Autodesk Inventor part; units mm, degrees
ref_plane "YZ Plane" through (0, 0, 0) normal (1, 0, 0) x (0, 1, 0)
ref_plane "XZ Plane" through (0, 0, 0) normal (0, 1, 0) x (-1, 0, 0)
ref_plane "XY Plane" through (0, 0, 0) normal (0, 0, 1) x (1, 0, 0)
sketch "Sketch1" plane through (0, 0, 0) normal (0, 1, 0) x (-1, 0, 0)
  line L0 (0, 0) -> (0, -32)
  line L1 (0, -32) -> (10.9556, -32)
  line L2 (10.9556, -32) -> (10.9556, 0)
  line L3 (10.9556, 0) -> (0, 0)
  dimension "d0" = 32
  dimension "d1" = 10.9556
extrude "Extrusion1" add sketch "Sketch1" along normal blind 2
sketch "Sketch2" plane through (-10.9556, 0, 0) normal (0, 0, 1) x (1, 0, 0)
  line L0 (10.9556, 0) -> (0, 0)
  line L1 (10.9556, 0) -> (9.9556, 0)
  line L2 (9.9556, 0) -> (9.9556, 2)
  line L3 (10.9556, 2) -> (0, 2)
  line L4 (10.9556, 2) -> (9.9556, 0)
  line L5 (0, 0) -> (0, 2)
  line L6 (0, 0) -> (1, 0)
  line L7 (1, 0) -> (0, 2)
  line L8 (1, 0) -> (0, 0)
  line L9 (0, 2) -> (0, 0)
  line L10 (0, 2) -> (10.9556, 2)
  line L11 (9.9556, 0) -> (1, 0)
  line L12 (9.9556, 0) -> (10.9556, 0)
  line L13 (10.9556, 0) -> (10.9556, 2)
  line L14 (10.9556, 2) -> (10.9556, 0)
  line L15 (10.9556, 0) -> (9.9556, 0)
  dimension "d4" = 1
  dimension "d5" = 1
extrude "Extrusion2" cut sketch "Sketch2" against normal through all contours L0 L4 L13 | L0 L5 L7
sketch "Sketch3" plane through (0, 2, 0) normal (0, 1, 0) x (1, 0, 0)
  line L0 (-10.9556, 32) -> (-10.9556, 0)
  line L1 (-10.9556, 32) -> (-10.9556, 0)
  line L2 (-10.9556, 0) -> (-10.9556, 16)
  line L3 (-10.9556, 16) -> (0, 16)
  line L4 (0, 0) -> (0, 32)
  line L5 (-10.9556, 0) -> (0, 0)
  line L6 (0, 32) -> (-10.9556, 32)
  line L7 (-10.9556, 32) -> (-10.9556, 30)
  line L8 (-10.9556, 28.5) -> (0, 28.5)
  line L9 (-10.9556, 0) -> (-10.9556, 2)
  line L10 (-10.9556, 3.5) -> (0, 3.5)
  line L11 (-10.9556, 30) -> (-10.9556, 22)
  line L12 (-10.9556, 20.5) -> (0, 20.5)
  line L13 (-10.9556, 2) -> (-10.9556, 10)
  line L14 (-10.9556, 11.5) -> (0, 11.5)
  line L15 (-10.9556, 20.5) -> (-11.494, 20.5)
  line L16 (-11.494, 20.5) -> (-11.494, 28.5)
  line L17 (-11.494, 28.5) -> (-10.9556, 28.5)
  line L18 (-11.494, 28.5) -> (-13.5464, 28.5)
  line L19 (-13.5464, 28.5) -> (-13.5464, 20.5)
  line L20 (-13.5464, 20.5) -> (-11.494, 20.5)
  line L21 (-11.494, 28.5) -> (-12.994, 28.5)
  line L22 (-11.494, 28.5) -> (-9.994, 28.5)
  line L23 (0, 30) -> (0, 22)
  line L24 (0, 20.5) -> (0.538, 20.5)
  line L25 (0.538, 20.5) -> (0.538, 28.5)
  line L26 (0.538, 28.5) -> (0, 28.5)
  line L27 (0.538, 28.5) -> (2.59, 28.5)
  line L28 (2.59, 28.5) -> (2.59, 20.5)
  line L29 (2.59, 20.5) -> (0.538, 20.5)
  line L30 (0.538, 28.5) -> (2.038, 28.5)
  line L31 (2.038, 28.5) -> (2.038, 20.5)
  line L32 (0.538, 28.5) -> (-0.962, 28.5)
  line L33 (-0.962, 30) -> (-0.962, 22)
  line L34 (-10.9556, 11.5) -> (-11.4936, 11.5)
  line L35 (-11.4936, 11.5) -> (-13.5456, 11.5)
  line L36 (-13.5456, 11.5) -> (-13.5456, 3.5)
  line L37 (-13.5456, 3.5) -> (-10.9556, 3.5)
  line L38 (0, 11.5) -> (0.538, 11.5)
  line L39 (0.538, 11.5) -> (2.59, 11.5)
  line L40 (2.59, 11.5) -> (2.59, 3.5)
  line L41 (2.59, 3.5) -> (0, 3.5)
  line L42 (0, 10) -> (0, 11.5)
  line L43 (0, 11.5) -> (-10.9556, 11.5)
  line L44 (0, 22) -> (0, 20.5)
  dimension "d8" = 32
  dimension "d10" = 2
  dimension "d11" = 2
  dimension "d12" = 8
  dimension "d13" = 8
  dimension "d14" = 0.5384
  dimension "d15" = 2.0524
  dimension "d16" = 1.5
  dimension "d17" = 1.5
  dimension "d23" = 0.538
  dimension "d24" = 2.052
  dimension "d25" = 1.5
  dimension "d26" = 1.5
  dimension "d27" = 0.538
  dimension "d28" = 2.052
  dimension "d29" = 0.538
  dimension "d43" = 1.5
  dimension "d44" = 1.5
extrude "Extrusion3" add sketch "Sketch3" along normal blind 4.4114 contours L8 L4 L12 L0 | L0 L15 L16 L17 | L16 L20 L19 L18 | L26 L25 L24 L4 | L27 L31 L29 L25 | L27 L28 L29 L31 | L14 L4 L10 L0 | L0 L37 L36 L35 L34 | L38 L39 L40 L41 L4
fillet "Fillet1" radius 2.2055 8 edges at (2.59, 6.4114, -7.5) (2.59, 2, -7.5) (2.59, 6.4114, -24.5) (2.59, 2, -24.5) (-13.5464, 6.4114, -24.5) (-13.5464, 2, -24.5) (-13.5456, 6.4114, -7.5) (-13.5456, 2, -7.5)
sketch "Sketch4" plane through (0, 6.4114, 0) normal (0, 1, 0) x (1, 0, 0)
  line L0 (-11.3401, 3.5) -> (-11.3401, 11.5)
  line L1 (-11.3401, 11.5) -> (-11.3401, 3.5)
  line L2 (-11.3401, 3.5) -> (-11.3401, 7.5)
  line L3 (-11.3401, 7.5) -> (-13.5456, 7.5)
  line L4 (-13.5456, 3.5) -> (-13.5456, 11.5)
  line L5 (-11.3401, 7.5) -> (2.59, 7.5)
  line L6 (2.59, 11.5) -> (2.59, 3.5)
  line L7 (0.3845, 3.5) -> (0.3845, 11.5)
  line L8 (-10.9556, 11.5) -> (0, 11.5)
  line L9 (-5.4778, 11.5) -> (-5.4778, 3.5)
  line L10 (-11.3401, 3.5) -> (0.3845, 3.5)
  line L11 (-5.4778, 7.5) -> (-6.9778, 7.5)
  line L12 (-6.9778, 7.5) -> (-5.4778, 11.5)
  line L13 (-5.4778, 7.5) -> (-3.9778, 7.5)
  line L14 (-3.9778, 7.5) -> (-5.4778, 3.5)
  line L15 (2.59, 2) -> (0.3845, 2)
  line L16 (-5.4778, 3.5) -> (2.59, 3.5)
  line L17 (2.59, 3.5) -> (2.59, 7.5)
  line L18 (-13.5456, 7.5) -> (-13.5456, 11.5)
  line L19 (-13.5456, 11.5) -> (-11.3401, 11.5)
  line L20 (-5.4778, 11.5) -> (-13.5456, 11.5)
  line L21 (-13.5456, 11.5) -> (-13.5456, 7.5)
  line L22 (-11.3409, 28.5) -> (-11.3409, 20.5)
  line L23 (-11.3409, 28.5) -> (-11.3409, 20.5)
  line L24 (-11.3409, 20.5) -> (-11.3409, 24.5)
  line L25 (-11.3409, 24.5) -> (0.3845, 24.5)
  line L26 (0.3845, 24.5) -> (-5.4782, 24.5)
  line L27 (-5.4782, 28.5) -> (-5.4782, 24.5)
  line L28 (-5.4782, 24.5) -> (-5.4782, 20.5)
  line L29 (-5.4782, 20.5) -> (-5.4782, 24.5)
  line L30 (-5.4782, 24.5) -> (-3.9782, 24.5)
  line L31 (-3.9782, 24.5) -> (-5.4782, 28.5)
  line L32 (-5.4782, 24.5) -> (-6.9782, 24.5)
  line L33 (-6.9782, 24.5) -> (-5.4782, 20.5)
  line L34 (-13.5464, 20.5) -> (-13.5464, 28.5)
  line L35 (-5.4782, 20.5) -> (-13.5464, 20.5)
  line L36 (-13.5464, 20.5) -> (-13.5464, 24.5)
  line L37 (-13.5464, 24.5) -> (-6.9782, 24.5)
  line L38 (-10.9556, 28.5) -> (0, 28.5)
  line L39 (-3.9782, 24.5) -> (4.3111, 24.5)
  line L40 (4.3111, 24.5) -> (4.3111, 28.5)
  line L41 (-5.4782, 28.5) -> (4.3111, 28.5)
  line L42 (0.3845, 28.5) -> (-11.3409, 28.5)
  point P0 (0, 0)
  point P1 (2.59, 10)
  point P2 (0.3845, 10)
  point P3 (0, 10)
  point P4 (0, 28.5)
  point P5 (-3.9782, 24.5)
  dimension "d33" = 1.5
  dimension "d34" = 1.5
  dimension "d37" = 1.5
  dimension "d38" = 1.5
extrude "Extrusion4" cut sketch "Sketch4" against normal blind 4.4114 contours L3 L4 L19 L0 | L0 L20 L8 L12 L5 | L14 L5 L7 L10 | L7 L5 L6 L16 | L25 L33 L35 L22 | L22 L35 L34 L37 | L38 L41 L40 L39 L25 L31
sketch "Sketch5" plane through (-3.9778, 6.4114, -7.5) normal (0, 0, 1) x (1, 0, 0)
  arc A0 (6.5678, -2.2055) -> (4.3623, 0) centre (4.3623, -2.2055) ccw
  line L0 (4.3623, 0) -> (4.3623, -2.2055)
  arc A1 (-7.3631, 0) -> (-9.5686, -2.2055) centre (-7.3631, -2.2055) ccw
  line L1 (-7.3631, 0) -> (-7.3631, -2.2055)
  circle A2 centre (-7.3631, -2.2055) radius 1.1
  circle A3 centre (4.3623, -2.2055) radius 1.1
  point P0 (3.9778, -6.4114)
  dimension "d39" = 2.2
  dimension "d40" = 2.2
extrude "Extrusion5" cut sketch "Sketch5" along normal through all both and the other way through all
sketch "Sketch6" plane through (0, 6.4114, 0) normal (0, 1, 0) x (1, 0, 0)
  point P0 (0, 0)
properties part number "pás-tiger I"
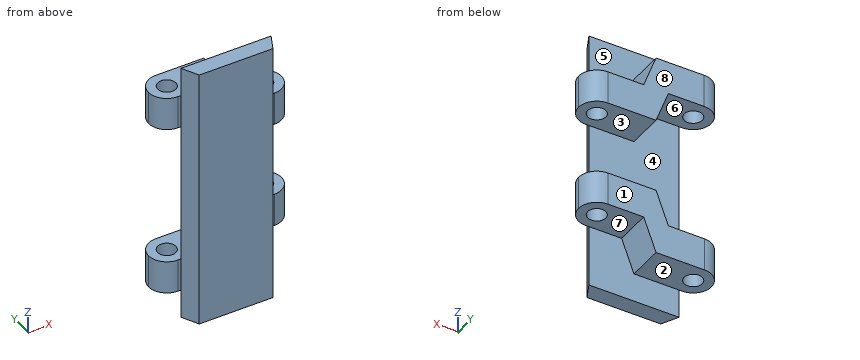
Part model, mm, in its own coordinate system. Face numbers are marked on the shaded views. A direction names the side the tool comes from. Coordinates: 2 decimals unless noted, no trailing zeros. Order: outer loops, then holes, each group sorted by start corner. A loop starts at its lowest first (then second) coordinate and runs counter-clockwise, first axis right, second up. Notation, with made-up numbers: (49, -8.5) -> (92, -8.5) arc R16 cw to (92, 0.5) -> close; hole circle Ø4 at (56, 48). An arc over 180 degrees is marked (long way). Put each result on its own line as item: value. Start each with the question number.
(1) Which spindle directions (+Z, -Z, +X, -X, +Y, -Y) get a long thin tool onto all of the face, cutting with end or side? Do the marked faces 5, 6, 7 and 8. Say none if no direction does.
(2) Band-saw the part on A-A (x = -8.75). Give the cut face in (y, z).
(3) Probe line 1 along Z through (x, y) = (-11, 5.75); line 2 along Z through (x, y) = (-1.5, 3); line 3 along Y through (x, z) = (-2.25, -13). List the from-to ranges inside material, lowest first. Write a range as [from, to].
(4) Band-saw the part on C-C (y = 3.5). Count the separate pieces of the cut face and the enclosed holes in it, then the cut area to 3 significant figures.
(5) Pin check, flat tips, straight feed: pin 1 Ø2 at (x, y) = (-3, 2) entering from +Z; pin 2 Ø3.5 at (x, z) = (-7, -19) entering from +Y; pin 3 Ø1.3 at (x, y) = (-8, 4) entering from -Z; pin 4 Ø3.5 at (x, y) = (-8.5, 4) entering from +Z. Stop position of each tip, or through.
(6) Band-saw the part on D-D (z = -12.5). Give the cut face in (x, y), then the cut area to 3 significant figures.
(7) Mould opens along Z. For the marked faces 1, 2, 3 and 4 say: pulls with the +Z half, pulls with the -Z half, needs draft (parallel to the pull), parting line crosses it, or undercut.
Determined:
1. face 5: +Z, +X, +Y
1. face 6: -X, +Y
1. face 7: -Z, +X, +Y
1. face 8: +Z, -Z, +X, -X, +Y
2. outline: (0, -32) -> (2, -32) -> (2, -28.5) -> (6.41, -28.5) -> (6.41, -24.5) -> (2, -24.5) -> (2, -7.5) -> (6.41, -7.5) -> (6.41, -3.5) -> (2, -3.5) -> (2, 0) -> (0, 0) -> close
3. line 1: z = [-28.5, -24.5], [-7.5, -3.5]
3. line 2: z = [-24.5, -20.5], [-11.5, -7.5]
3. line 3: y = [0, 2]
4. separate pieces: 6
4. enclosed holes: 0
4. area: 112 mm²
5. pin 1: stops at z = 0
5. pin 2: stops at y = 2
5. pin 3: stops at z = -28.5
5. pin 4: stops at z = -3.5
6. outline: (-10.96, 2) -> (-9.96, 0) -> (-1, 0) -> (0, 2) -> close
6. area: 19.9 mm²
7. face 1: needs draft
7. face 2: pulls with the -Z half
7. face 3: undercut
7. face 4: undercut
